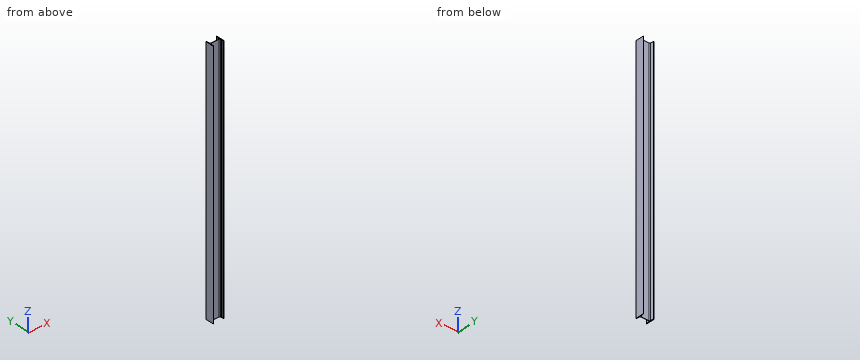
```python
from build123d import *

# Parameters (mm, degrees)
BOSS_EXTRUDE1_DEPTH = 3700
SCALE1_SCALE        = 0.75


with BuildPart() as part:
    # Sketch1 → Boss-Extrude1 (new body)
    with BuildSketch(Plane.XY.offset(1800)):
        with BuildLine():
            Line((129, 60.46884946), (129, 30))
            Line((129, 30), (124.919748757, 30))
            Line((124.919748757, 30), (122.792728308, 12.689402566))
            ThreePointArc((122.792728308, 12.689402566), (119.171200489, 5.771495525), (111.871083085, 3))
            Line((111.871083085, 3), (-1.871083085, 3))
            ThreePointArc((-1.871083085, 3), (-9.171200492, 5.771495528), (-12.792728309, 12.689402573))
            Line((-12.792728309, 12.689402573), (-18.294338419, 58.536153493))
            ThreePointArc((-18.294338419, 58.536153493), (-19.775872526, 61.366206375), (-22.762284192, 62.5))
            Line((-22.762284192, 62.5), (-25, 62.5))
            Line((-25, 62.5), (-25, -62.5))
            Line((-25, -62.5), (-22.762284192, -62.5))
            ThreePointArc((-22.762284192, -62.5), (-19.775872526, -61.366206375), (-18.294338419, -58.536153493))
            Line((-18.294338419, -58.536153493), (-12.792728309, -12.689402573))
            ThreePointArc((-12.792728309, -12.689402573), (-9.171200492, -5.771495528), (-1.871083085, -3))
            Line((-1.871083085, -3), (111.871083085, -3))
            ThreePointArc((111.871083085, -3), (119.171200492, -5.771495528), (122.792728309, -12.689402573))
            Line((122.792728309, -12.689402573), (124.87, -30))
            Line((124.87, -30), (129, -30))
            Line((129, -30), (129, -60.46884946))
            ThreePointArc((129, -60.46884946), (130.62450761, -61.959786773), (132.762284192, -62.5))
            Line((132.762284192, -62.5), (135, -62.5))
            Line((135, -62.5), (135, 62.5))
            Line((135, 62.5), (132.762284192, 62.5))
            ThreePointArc((132.762284192, 62.5), (130.62450761, 61.959786773), (129, 60.46884946))
        make_face()
    extrude(amount=-BOSS_EXTRUDE1_DEPTH)


with BuildPart() as part_1:
    # Scale1: scaled about (51.838667986, -0.00324275, -50)
    add(part.part.scale(SCALE1_SCALE).moved(Location((12.959666996, -0.000810687, -12.5))))


solid = part_1.part
```
Here's how the part is built. I have some questions about the finished solid (model axes, mm). Coordinates: 2 decimals unless noted, no trailing zeros. Loops run counter-clockwise (first coordinate to the right, second up) from the corner with the lowest first, then second, coordinate; pieces in that order, holes last. Notation, with made-up numbers: (48, -12) - (98, -12) arc R30 ccw to (98, 24) - close; hole circle Ø8 at (-15, -6). An arc over 180 degrees is marked (long way). Answer as CSV lines item,"result".
Q1. If I drill on L1, parallel to X at y = 41, z = -469.5; L2, parallel to X at y = -12.5, z = -911.5; L3, parallel to Y at x = 53, z = -1273.5, over which ranges is the centre line in solid material (lowest first)? Write a range as [from, to].
Response:
L1,"[-5.79, -0.41], [109.71, 114.21]"
L2,"[-5.79, 3.01], [105.41, 114.21]"
L3,"[-2.25, 2.25]"
Q2. If we section it at A-A, the plane z = -182.5: Write out the boundary of the cut face in (x, y) (3 decimals), and give its area (3 significant figures).
Response:
outline,"(-5.79, -46.876) - (-4.112, -46.876) arc R3.375 ccw to (-0.761, -43.903) - (3.365, -9.518) arc R8.25 cw to (11.556, -2.251) - (96.863, -2.251) arc R8.25 cw to (105.054, -9.518) - (106.612, -22.501) - (109.71, -22.501) - (109.71, -45.352) arc R3.375 ccw to (112.531, -46.876) - (114.21, -46.876) - (114.21, 46.874) - (112.531, 46.874) arc R3.375 ccw to (109.71, 45.351) - (109.71, 22.499) - (106.649, 22.499) - (105.054, 9.516) arc R8.25 cw to (96.863, 2.249) - (11.556, 2.249) arc R8.25 cw to (3.365, 9.516) - (-0.761, 43.901) arc R3.375 ccw to (-4.112, 46.874) - (-5.79, 46.874) - close"
area,"1,810 mm2"
Q3. If we section it at B-B, the plane x = 78: Write out the boundary of the cut face in (y, z).
Response:
outline,"(-2.25, -1437.5) - (2.25, -1437.5) - (2.25, 1337.5) - (-2.25, 1337.5) - close"
Q4. For pin 1 (2 mm diameter, centred on x = 61.5, z = 323.5, fed in from +Y); pin 2 (1.5 mm diameter, centred on x = 107.5, z = 75, fed in from -Y); pin 3 (0.9 mm diameter, centred on x = 107.5, z = 625, fed in from +Y), each with a flat end and sliding along its axis, tell me the tip position at first contact or that it passes through.
Response:
pin 1,"y = 2.25"
pin 2,"y = -22.5"
pin 3,"y = 22.5"
